For this review, use the dimensioned drawing (mm, ordinates from the lowest corner) and the shaded views. A direction names the side the tool comes from. Give positions to 0.01 mm unless a question says otherwise; leave off trailing zeros. Loops run counter-clockwise (first coordinate to the right, second up) from the corner with the lowest first, then second, coordinate; pieces in that order, holes last. Notation, with made-up numbers: M -27,37 L 11,37 A26 cw 11,53 Z; hole C 30.25,50.25 d11. An arc over 180 degrees is marked long. Use one line per item in the form item = value. Start each with the question number.
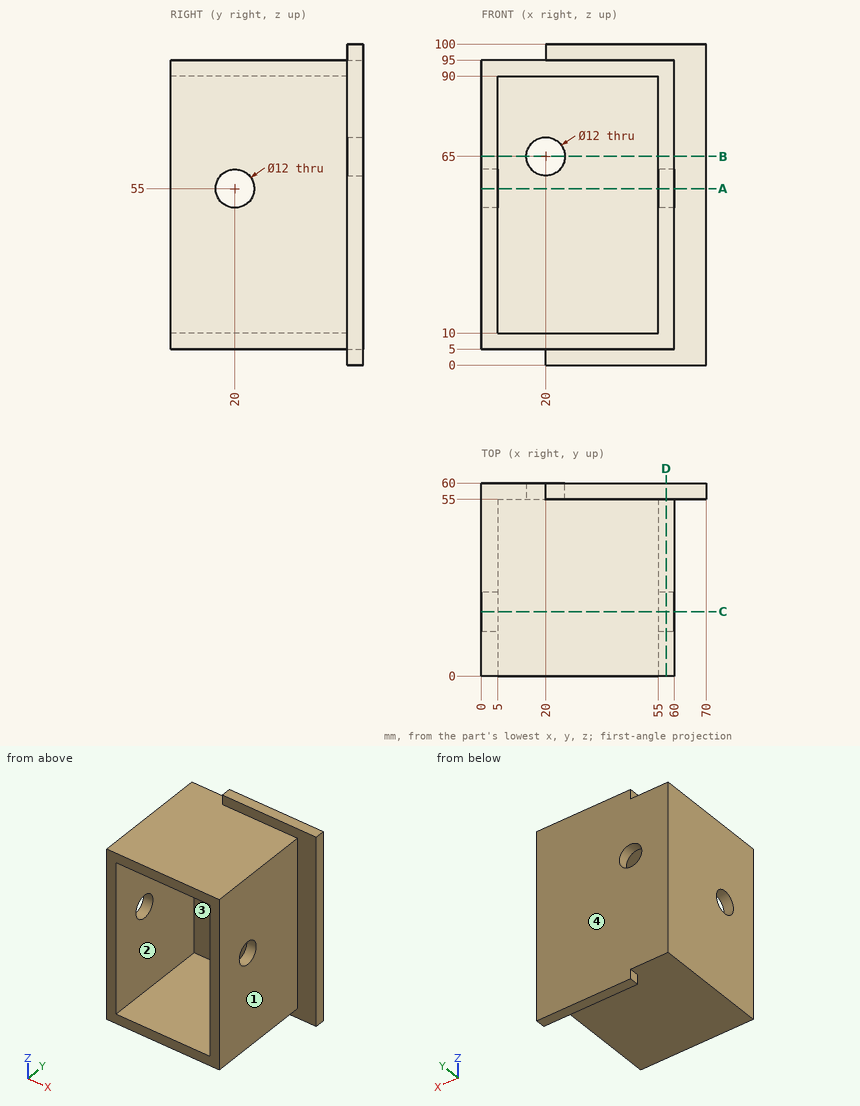
Q1. Take a section at C-C on y = 20. Give the boundary of the cut face in (x, z).
Q2. For the marked faces 3 and 4, list the 3-axis set-ups (+Z, -Z, +X, -X, +Y, -Y) from which the entire face can be reached by the end or side of a thin tool; tool diameter is ignored.
Q3. The part is to be moulded in two halves that separate along Z. For the marked faces 1 and 2, say which applies: pulls with the +Z half, pulls with the -Z half, needs draft (parallel to the pull), parting line crosses it, or undercut.
Q4. Take a section at A-A on z = 55. Give the boundary of the cut face in (x, y), plus the area to 3 significant figures.
Q5. Wall thickness on probe 1 along X at (y, z) = (36, 25.5); probe 2 along Z at (x, y) = (58.8, 20); probe 3 along Z at (x, y) = (44.5, 36): over which ranges is each line inside the solid? List them lowest first.
Q6. Clearance check with flat-ended pins moving along their axes: pin 1 Ø2 at (x, z) = (10, 75) entering from -Y; pin 2 Ø16.5 at (y, z) = (19, 71) entering from +X; pin 3 Ø1 at (x, y) = (28.5, 32.5) entering from -Z. State where each tip first meets the part, or that it passes through.
Q7. Take a section at B-B on z = 65. Give the boundary of the cut face in (x, y).
Q8. Take a section at D-D on x = 57.5. Give the boundary of the cut face in (y, z).
Response values:
q1.outline = M 0,5 L 60,5 L 60,49 L 55,49 L 55,10 L 5,10 L 5,49 L 0,49 Z; M 0,61 L 5,61 L 5,90 L 55,90 L 55,61 L 60,61 L 60,95 L 0,95 Z
q2.face_3 = -Y
q2.face_4 = +Z, -Z, +X, -X, +Y
q3.face_1 = needs draft
q3.face_2 = undercut
q4.outline = M 0,0 L 5,0 L 5,14 L 0,14 Z; M 0,26 L 5,26 L 5,55 L 55,55 L 55,26 L 60,26 L 60,55 L 70,55 L 70,60 L 0,60 Z; M 55,0 L 60,0 L 60,14 L 55,14 Z
q4.area = 780 mm^2
q5.probe_1 = 0 to 5, 55 to 60
q5.probe_2 = 5 to 49, 61 to 95
q5.probe_3 = 5 to 10, 90 to 95
q6.pin_1 = 55
q6.pin_2 = 60
q6.pin_3 = 5
q7.outline = M 0,0 L 5,0 L 5,55 L 14,55 L 14,60 L 0,60 Z; M 26,55 L 55,55 L 55,0 L 60,0 L 60,55 L 70,55 L 70,60 L 26,60 Z
q8.outline = M 0,5 L 55,5 L 55,0 L 60,0 L 60,100 L 55,100 L 55,95 L 0,95 Z; hole C 20,55 d12
